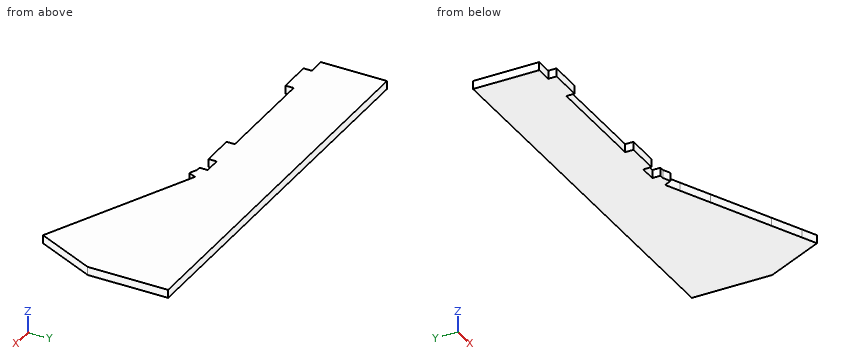
Autodesk Inventor part; units mm, degrees
ref_plane "YZ Plane" through (0, 0, 0) normal (1, 0, 0) x (0, 1, 0)
ref_plane "XZ Plane" through (0, 0, 0) normal (0, 1, 0) x (-1, 0, 0)
ref_plane "XY Plane" through (0, 0, 0) normal (0, 0, 1) x (1, 0, 0)
sketch "Sketch1" plane through (0, 0, 0) normal (0, 0, 1) x (1, 0, 0)
  line L0 (0, 0) -> (0, 25.4)
  line L1 (0, 25.4) -> (79.375, 25.4)
  line L2 (79.375, 25.4) -> (79.375, 0)
  line L3 (79.375, 0) -> (73.025, 0)
  line L4 (73.025, 0) -> (73.025, -3.175)
  line L5 (73.025, -3.175) -> (60.325, -3.175)
  line L6 (60.325, -3.175) -> (60.325, 0)
  line L7 (0, 0) -> (6.35, 0)
  line L8 (6.35, 0) -> (6.35, -3.175)
  line L9 (6.35, -3.175) -> (19.05, -3.175)
  line L10 (19.05, -3.175) -> (19.05, 0)
  line L11 (19.05, 0) -> (60.325, 0)
  dimension "d0" = 25.4
  dimension "d1" = 79.375
  dimension "d2" = 6.35
  dimension "d4" = 3.175
  dimension "d5" = 12.7
  dimension "d6" = 6.35
  dimension "d7" = 3.175
  dimension "d8" = 12.7
  dimension "d9" = 25.4
  dimension "d10" = 25.4
extrude "Extrusion1" add sketch "Sketch1" along normal blind 3.175
sketch "Sketch2" plane through (0, 0, 3.175) normal (0, 0, 1) x (1, 0, 0)
  line L0 (141.5184, -31.3531) -> (142.8602, -28.4755)
  line L1 (125.5951, -20.4247) -> (137.1052, -25.7919)
  line L2 (124.2533, -23.3022) -> (125.5951, -20.4247)
  line L3 (135.7634, -28.6694) -> (124.2533, -23.3022)
  line L4 (137.1052, -25.7919) -> (135.7634, -28.6694)
  line L5 (101.233, -12.5677) -> (89.7229, -7.2004)
  line L6 (102.5748, -9.6902) -> (101.233, -12.5677)
  line L7 (91.0647, -4.3229) -> (102.5748, -9.6902)
  line L8 (89.7229, -7.2004) -> (91.0647, -4.3229)
  line L9 (83.9679, -4.5168) -> (85.3097, -1.6393)
  line L10 (79.375, 0) -> (79.375, -3.175)
  line L11 (79.375, -3.175) -> (81.0903, -3.175)
  line L12 (83.9679, -4.5168) -> (81.0903, -3.175)
  line L13 (79.375, -3.175) -> (79.375, 25.4)
  line L14 (79.375, 25.4) -> (87.4253, 25.4)
  line L15 (83.9679, -4.5168) -> (85.3097, -1.6393)
  line L16 (85.3097, -1.6393) -> (91.0647, -4.3229)
  line L17 (91.0647, -4.3229) -> (89.7229, -7.2004)
  line L18 (89.7229, -7.2004) -> (101.233, -12.5677)
  line L19 (102.5748, -9.6902) -> (101.233, -12.5677)
  line L20 (102.5748, -9.6902) -> (125.5951, -20.4247)
  line L21 (125.5951, -20.4247) -> (124.2533, -23.3022)
  line L22 (124.2533, -23.3022) -> (135.7634, -28.6694)
  line L23 (137.1052, -25.7919) -> (135.7634, -28.6694)
  line L24 (142.8602, -28.4755) -> (137.0616, -25.7716)
  line L25 (142.8602, -28.4755) -> (153.5947, -5.4553)
  line L26 (79.375, 25.4) -> (0, 25.4)
  line L27 (87.4253, 25.4) -> (153.5947, 25.4)
  line L28 (153.5947, 25.4) -> (153.5947, -5.4553)
  dimension "d13" = 25.4
extrude "Extrusion2" add sketch "Sketch2" against normal blind 3.175 contours L20 L7 L16 L9 L12 L11 L10 L13 L14 L27 L28 L25 L24 L1
properties part number "Side Wall" material "Polycarbonate, Clear"
Model file for the job. Use its own axes, mm. Coordinates: 2 decimals unless noted, no trailing zeros. Loops run counter-clockwise (first coordinate to the right, second up) from the corner with the lowest first, then second, coordinate; pieces in that order, holes last. Notation, with made-up numbers: (7.25, -3) -> (64.25, -3) arc R11 ccw to (64.25, 1) -> close; hole circle Ø7 at (10, 13). An arc over 180 degrees is marked (long way). Answer as a JSON object with one key per item and string values.
Q1. Cut at A-A (x = 13.5). List the corners of the cut face in (y, z) (3 decimals), and give its area (3 significant figures).
Report:
{"outline": "(-3.175, 0) -> (25.4, 0) -> (25.4, 3.175) -> (-3.175, 3.175) -> close", "area": "90.7 mm2"}
Q2. Flat gauge pins, fed straight in: P1, Ø1, axis at x = 65.5, z = 1.5, coming from the -Y side (3 decimals); P2, Ø1, axis at y = -1.5, z = 2, coming from the -X side; P3, Ø1, axis at y = -4, z = 2, coming from the -X side. Where does each tip first touch, or does it go through?
Report:
{"P1": "stops at y = -3.175", "P2": "stops at x = 6.35", "P3": "stops at x = 81.79"}
Q3. Cut at C-C (y = -23). List the corners of the cut face in (x, z) (3 decimals), and give its area (3 significant figures).
Report:
{"outline": "(131.118, 0) -> (145.413, 0) -> (145.413, 3.175) -> (131.118, 3.175) -> close", "area": "45.4 mm2"}
Q4. Probe probe 1 along Y at (x, z) = (25, 2.6); probe 2 along Y at (x, z) = (15, 1.7) (3 decimals); probe 3 along X at (y, z) = (-5.5, 1.35). List the from-to ranges inside material, lowest first.
Report:
{"probe 1": "y = 0 to 25.4", "probe 2": "y = -3.175 to 25.4", "probe 3": "x = 93.59 to 153.57"}
